from build123d import *

# Parameters (mm, degrees)
SKETCH1_W           = 3
SKETCH1_H           = 16
SKETCH1_R           = 12.5
SKETCH1_R_2         = 8
BOSS_EXTRUDE1_DEPTH = 3
SKETCH2_W           = 40
SKETCH2_H           = 1.6
BOSS_EXTRUDE2_DEPTH = 3


with BuildPart() as part:
    # Sketch1 → Boss-Extrude1 (new body)
    with BuildSketch(Plane(origin=(0, 0, 0), x_dir=(0, 0, -1), z_dir=(1, 0, 0))):
        Polygon((125, -40), (180, -8), (180, -3), (146.666666667, -3), (146.666666667, 0), (106.666666667, 0), (106.666666667, -3), (73.333333333, -3), (73.333333333, 0), (33.333333333, 0), (33.333333333, -3), (0, -3), (0, 0), (-4, 0), (-4, -40), (0, -40), align=None)
        with Locations((1.5, -20)):
            Rectangle(SKETCH1_W, SKETCH1_H, mode=Mode.SUBTRACT)
        with Locations((23, -20)):
            Circle(SKETCH1_R, mode=Mode.SUBTRACT)
        with Locations((54.5, -20)):
            Circle(SKETCH1_R, mode=Mode.SUBTRACT)
        with Locations((86, -20)):
            Circle(SKETCH1_R, mode=Mode.SUBTRACT)
        with Locations((117.5, -20)):
            Circle(SKETCH1_R, mode=Mode.SUBTRACT)
        with Locations((145, -14)):
            Circle(SKETCH1_R_2, mode=Mode.SUBTRACT)
    extrude(amount=BOSS_EXTRUDE1_DEPTH)

    # Sketch2 → Boss-Extrude2 (add)
    with BuildSketch(Plane(origin=(3, 0, 0), x_dir=(0, 0, -1), z_dir=(1, 0, 0))):
        with Locations((126.666666667, 0.8)):
            Rectangle(SKETCH2_W, SKETCH2_H)
    extrude(amount=-BOSS_EXTRUDE2_DEPTH)


solid = part.part
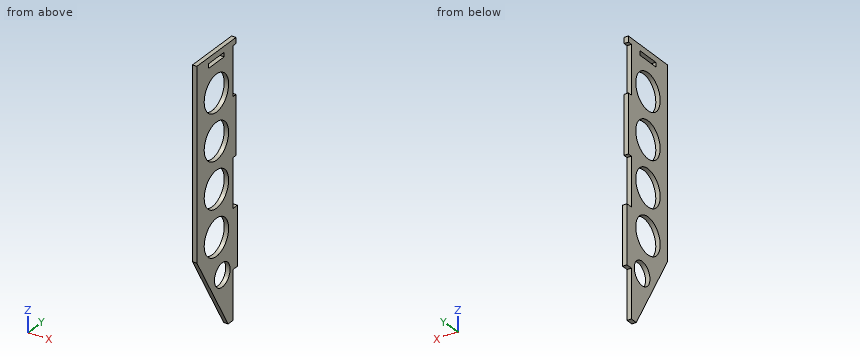
The model under review builds one solid part; all positions refer to its coordinate system, in mm. Coordinates: 2 decimals unless noted, no trailing zeros. Loops run counter-clockwise (first coordinate to the right, second up) from the corner with the lowest first, then second, coordinate; pieces in that order, holes last.
(1) Consider section C-C, the plane x = 2.1. Give the boundary of the cut face in (y, z), plus the area to 3 significant figures.
Determined:
outline: (-40, -125) - (-8, -180) - (-3, -180) - (-3, -146.67) - (1.6, -146.67) - (1.6, -106.67) - (-3, -106.67) - (-3, -73.33) - (0, -73.33) - (0, -33.33) - (-3, -33.33) - (-3, 0) - (0, 0) - (0, 4) - (-40, 4) - close; hole circle Ø25 at (-20, -117.5); hole circle Ø25 at (-20, -86); hole circle Ø25 at (-20, -54.5); hole circle Ø25 at (-20, -23); hole (-28, -3) - (-12, -3) - (-12, 0) - (-28, 0) - close; hole circle Ø16 at (-14, -145)
area: 4,030 mm2
(2) Consider section D-D, the plane z = -23. Give the boundary of the cut face in (x, y).
Determined:
outline: (0, -40) - (3, -40) - (3, -32.5) - (0, -32.5) - close; (0, -7.5) - (3, -7.5) - (3, -3) - (0, -3) - close
(3) Consider section B-B, the plane y = -14. Give the boundary of the cut face in (x, z).
Determined:
outline: (0, -169.69) - (3, -169.69) - (3, -153) - (0, -153) - close; (0, -137) - (3, -137) - (3, -128.47) - (0, -128.47) - close; (0, -106.53) - (3, -106.53) - (3, -96.97) - (0, -96.97) - close; (0, -75.03) - (3, -75.03) - (3, -65.47) - (0, -65.47) - close; (0, -43.53) - (3, -43.53) - (3, -33.97) - (0, -33.97) - close; (0, -12.03) - (3, -12.03) - (3, -3) - (0, -3) - close; (0, 0) - (3, 0) - (3, 4) - (0, 4) - close
(4) Insertion check: P1, Ø0.9, axis at x = 2, y = -0.5, coming from the -Z side; P2, Ø0.9, axis at x = 1, z = -93.5, coming from the +Y side; P3, Ø1, axis at x = 0.5, z = -130.5, coming from the -Y side; P4, Ø15, axis at y = -20, z = -23, coming from the +X side. Each pin has a flat end and moves straight along its axis. Give the tip position at first contact, or say it passes through.
Determined:
P1: stops at z = -146.67
P2: stops at y = -3
P3: stops at y = -37.09
P4: passes through
(5) Wall thickness on L1, parallel to Y at x = 0.75, z = -86; L2, parallel to Z at x = 1.7, y = -23; L3, parallel to Z at x = 1.1, y = -9 (3 decimals): over which ranges is each line inside the solid? List them lowest first.
Determined:
L1: y = -40 to -32.5, -7.5 to -3
L2: z = -154.22 to -129.63, -105.37 to -98.13, -73.87 to -66.63, -42.37 to -35.13, -10.87 to -3, 0 to 4
L3: z = -178.281 to -151.245, -138.755 to -123.437, -111.563 to -91.937, -80.063 to -60.437, -48.563 to -28.937, -17.063 to 4
(6) Consider section A-A, the plane z = -117.5. Give the boundary of the cut face in (x, y), plus the area to 3 significant figures.
Determined:
outline: (0, -40) - (3, -40) - (3, -32.5) - (0, -32.5) - close; (0, -7.5) - (3, -7.5) - (3, 1.6) - (0, 1.6) - close
area: 49.8 mm2
